Geometry check sheet. Reference: drawing and pictorial views, mm from the part's lowest x, y, z. A direction names the side the tool comes from. Coordinates: 2 decimals unless noted, no trailing zeros. Loops run counter-clockwise (first coordinate to the right, second up) from the corner with the lowest first, then second, coordinate; pieces in that order, holes last. Notation, with made-up numbers: (49, 3) -> (95, 3) arc R26 cw to (95, 32) -> close; hole circle Ø6 at (-39.5, -15.5). An arc over 180 degrees is marked (long way). Answer as a JSON object with one key per item and string values. Group by question number.
Q1. Cross-section at D-D on x = 14. Record the boundary of the cut face in (y, z) (1 decimal).
Q2. Gauge pin test, flat ends, axial feed: pin 1 Ø4 at (x, z) = (23.75, 21) entering from +Y; pin 2 Ø2 at (y, z) = (21, 5.5) entering from +X. Record the tip position at first contact, or that the pin passes through.
Q3. Release check for a two-part mould opening along Y. For the marked faces 1, 2, 3 and 4 record: released by +Y, released by -Y, zero draft, split by the parting line, or undercut.
Q4. Scan lines: L1, parallel to X at y = 2.4, z = 5; L2, parallel to Z at x = 23, y = 2; L3, parallel to X at y = 20, z = 17.75. Record each from-to range of solid material in increasing order.
Q5. Cross-section at C-C on z = 5. Give the number of separate pieces and of enclosed holes in the cut face, and give its area (3 significant figures).
Q6. Set-up check for the marked faces 5 and 6: record each of +Z, -Z, +X, -X, +Y, -Y from which the full face is reachable in a straight line by a thin tool's end or side.
Q7. Cross-section at B-B on z = 15.25. Record the boundary of the cut face in (x, y) (1 decimal).
Q8. Cross-section at A-A on x = 23.75. Record the boundary of the cut face in (y, z).
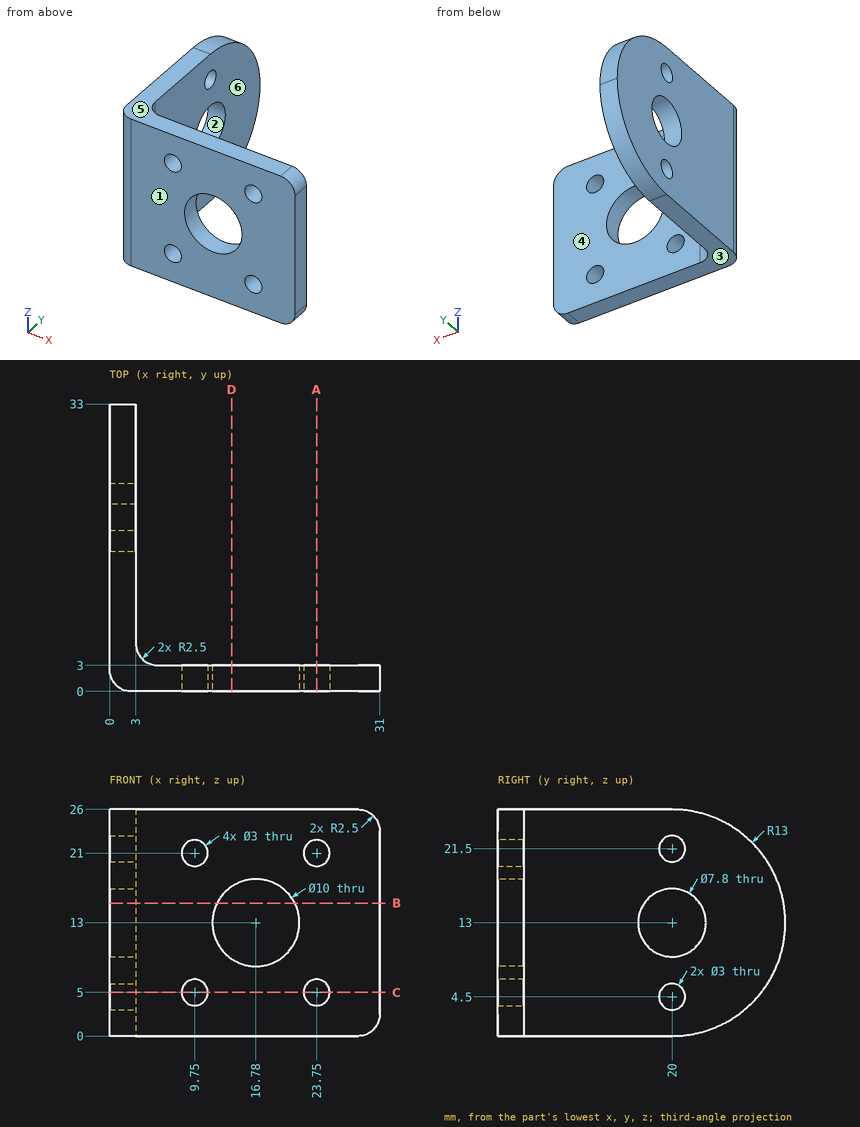
Computed values:
{
 "1": {"outline": "(0, 0) -> (3, 0) -> (3, 8.8) -> (0, 8.8) -> close; (0, 17.2) -> (3, 17.2) -> (3, 26) -> (0, 26) -> close"},
 "2": {"pin 1": "stops at y = 3", "pin 2": "stops at x = 3"},
 "3": {"face 1": "released by -Y", "face 2": "undercut", "face 3": "zero draft", "face 4": "released by +Y"},
 "4": {"L1": "x = 0 to 8.25, 11.25 to 22.25, 25.25 to 31", "L2": "z = 0 to 3.7, 6.3 to 19.7, 22.3 to 26", "L3": "x = 0 to 3"},
 "5": {"separate pieces": "4", "enclosed holes": "0", "area": "148 mm²"},
 "6": {"face 5": "+Z, +X, -X, +Y, -Y", "face 6": "+Z, -Z, +X, +Y"},
 "7": {"outline": "(0, 2.5) arc R2.5 ccw to (2.5, 0) -> (12.3, 0) -> (12.3, 3) -> (5.5, 3) arc R2.5 cw to (3, 5.5) -> (3, 16.8) -> (0, 16.8) -> close; (0, 23.2) -> (3, 23.2) -> (3, 32.8) -> (0, 32.8) -> close; (21.2, 0) -> (31, 0) -> (31, 3) -> (21.2, 3) -> close"},
 "8": {"outline": "(0, 0) -> (3, 0) -> (3, 3.5) -> (0, 3.5) -> close; (0, 6.5) -> (3, 6.5) -> (3, 19.5) -> (0, 19.5) -> close; (0, 22.5) -> (3, 22.5) -> (3, 26) -> (0, 26) -> close"}
}
